Build history of the part. All positions in model axes, mm. Round coordinates to 2 decimals unless told otherwise and drop trailing zeros. Use a Markdown table: item, result.
from build123d import *

# Parameters (mm, degrees)
SKETCH1_W           = 124.35
SKETCH1_H           = 33
BOSS_EXTRUDE1_DEPTH = 3.175
SKETCH2_W           = 9.65
SKETCH2_H           = 2.8
SKETCH2_H_2         = 3
CUT_EXTRUDE1_DEPTH  = 65.405444257
SKETCH4_W           = 2.8
SKETCH4_H           = 3
SKETCH4_W_2         = 6.175
SKETCH4_H_2         = 15
CUT_EXTRUDE2_DEPTH  = 65.405444257
SKETCH6_W           = 3
SKETCH6_H           = 1.375
CUT_EXTRUDE3_DEPTH  = 65.405444257
CUT_SWEEP1_DEPTH    = 3.175
SKETCH12_R          = 0.75
CUT_EXTRUDE6_DEPTH  = 65.405444385
CUT_EXTRUDE7_DEPTH  = 65.405444385
FILLET6_R           = 2
FILLET7_R           = 0.5
SKETCH14_W          = 20
SKETCH14_H          = 16
CUT_EXTRUDE8_DEPTH  = 65.405444385
FILLET8_R           = 0.5


# Read off the part's stored shape, not the designer's step: Cut-Sweep1
with BuildPart() as part:
    # Sketch1 → Boss-Extrude1 (new body)
    with BuildSketch(Plane.XY):
        Rectangle(SKETCH1_W, SKETCH1_H)
    extrude(amount=BOSS_EXTRUDE1_DEPTH)

    # Sketch2 → Cut-Extrude1 (cut, through all)
    with BuildSketch(Plane.XY.offset(3.175)):
        with Locations((-25, -13.1)):
            Rectangle(SKETCH2_W, SKETCH2_H)
        with Locations((25, -13.1)):
            Rectangle(SKETCH2_W, SKETCH2_H)
        with Locations((-25, 15)):
            Rectangle(SKETCH2_W, SKETCH2_H_2)
        with Locations((25, 15)):
            Rectangle(SKETCH2_W, SKETCH2_H_2)
    extrude(amount=-CUT_EXTRUDE1_DEPTH, mode=Mode.SUBTRACT)

    # Sketch4 → Cut-Extrude2 (cut, through all)
    with BuildSketch(Plane.XY.offset(3.175)):
        with Locations((-57.775, 15)):
            Rectangle(SKETCH4_W, SKETCH4_H)
        with Locations((-59.0875, 0)):
            Rectangle(SKETCH4_W_2, SKETCH4_H_2)
        with Locations((-57.775, -15)):
            Rectangle(SKETCH4_W, SKETCH4_H)
        with Locations((57.775, 15)):
            Rectangle(SKETCH4_W, SKETCH4_H)
        with Locations((59.0875, 0)):
            Rectangle(SKETCH4_W_2, SKETCH4_H_2)
        with Locations((57.775, -15)):
            Rectangle(SKETCH4_W, SKETCH4_H)
    extrude(amount=-CUT_EXTRUDE2_DEPTH, mode=Mode.SUBTRACT)

    # Sketch6 → Cut-Extrude3 (cut, through all)
    with BuildSketch(Plane.XY.offset(3.175)):
        with Locations((-60.675, 15.8125)):
            Rectangle(SKETCH6_W, SKETCH6_H)
        with Locations((-60.675, -15.8125)):
            Rectangle(SKETCH6_W, SKETCH6_H)
        with Locations((60.675, 15.8125)):
            Rectangle(SKETCH6_W, SKETCH6_H)
        with Locations((60.675, -15.8125)):
            Rectangle(SKETCH6_W, SKETCH6_H)
    extrude(amount=-CUT_EXTRUDE3_DEPTH, mode=Mode.SUBTRACT)

    # Cut-Sweep1 outline → Cut-Sweep1 (cut)
    with BuildSketch(Plane.XY):
        with BuildLine():
            add(Edge.make_bspline(
                [(-56, -6), (-55.016272395, -6.040912607), (-53.484317245, -6.110006936), (-52.10462272, -6.208217255), (-51.370216858, -6.312882143), (-50.849013323, -6.424427059), (-50.274077583, -6.562740427), (-49.507561658, -6.770408498), (-47.98416767, -7.234467607), (-46.535590196, -7.742954919), (-44.899823838, -8.383891144), (-43.265010906, -9.091671777), (-41.074137026, -10.055384808), (-38.357692762, -10.850187014), (-36.1078612, -11.027108547), (-34.793437631, -10.999002823)],
                knots=[0, 0, 0, 0, 0.052266667, 0.104533333, 0.1568, 0.188540911, 0.209066667, 0.261333333, 0.3136, 0.4368, 0.46346514, 0.56, 0.706666667, 0.853333333, 1, 1, 1, 1], degree=3))
            Line((-56, -6), (-56, -7.5))
            add(Edge.make_bspline(
                [(-56, -7.5), (-55.020423649, -7.540842864), (-53.496771007, -7.609797709), (-52.171479553, -7.70829789), (-51.569513747, -7.80075633), (-51.115986388, -7.900930823), (-50.592043829, -8.028791809), (-49.863497697, -8.22781936), (-48.398796638, -8.676488924), (-46.992197023, -9.172450468), (-45.412650318, -9.7933523), (-43.831176536, -10.480660701), (-41.561928867, -11.478467634), (-38.556226285, -12.350501385), (-36.110914304, -12.525218982), (-34.698750526, -12.49601129)],
                knots=[0, 0, 0, 0, 0.052266667, 0.104533333, 0.1568, 0.188540911, 0.209066667, 0.261333333, 0.3136, 0.4368, 0.46346514, 0.56, 0.706666667, 0.853333333, 1, 1, 1, 1], degree=3))
            Line((-34.698750526, -12.49601129), (-34.793437631, -10.999002823))
        make_face()
    cut_sweep1 = extrude(amount=CUT_SWEEP1_DEPTH, mode=Mode.SUBTRACT)

    # Mirror1: Cut-Sweep1 across plane
    add(cut_sweep1.mirror(Plane.ZY), mode=Mode.SUBTRACT)

    # Sketch12 → Cut-Extrude6 (cut, through all)
    with BuildSketch(Plane.XY.offset(3.175)):
        with Locations((-34.746094079, -11.747507056)):
            Circle(SKETCH12_R)
        with Locations((34.746094079, -11.747507056)):
            Circle(SKETCH12_R)
    extrude(amount=-CUT_EXTRUDE6_DEPTH, mode=Mode.SUBTRACT)

    # Sketch13 → Cut-Extrude7 (cut, through all)
    with BuildSketch(Plane.XY.offset(3.175)):
        Polygon((-56, 7.5), (-62.175, 11.3125), (-62.175, 7.5), align=None)
        Polygon((-56, -7.5), (-62.175, -11.3125), (-62.175, -7.5), align=None)
        Polygon((56, 7.5), (62.175, 11.3125), (62.175, 7.5), align=None)
        Polygon((56, -7.5), (62.175, -11.3125), (62.175, -7.5), align=None)
    extrude(amount=-CUT_EXTRUDE7_DEPTH, mode=Mode.SUBTRACT)

    # Fillet6
    fillet6_edges = [part.edges().sort_by_distance(p)[0] for p in [
        (62.175, -15.125, 1.5875),
        (62.175, -11.3125, 1.5875),
        (56, -7.5, 1.5875),
        (56, 7.5, 1.5875),
        (62.175, 11.3125, 1.5875),
        (62.175, 15.125, 1.5875),
        (-62.175, -15.125, 1.5875),
        (-62.175, -11.3125, 1.5875),
        (-56, -7.5, 1.5875),
        (-62.175, 15.125, 1.5875),
        (-62.175, 11.3125, 1.5875),
        (-56, 7.5, 1.5875),
    ]]
    fillet(fillet6_edges, radius=FILLET6_R)

    # Fillet7
    fillet7_edges = [part.edges().sort_by_distance(p)[0] for p in [
        (59.175, 15.125, 1.5875),
        (59.175, -15.125, 1.5875),
        (-59.175, -15.125, 1.5875),
        (-59.175, 15.125, 1.5875),
        (20.175, 16.5, 1.5875),
        (29.825, 16.5, 1.5875),
        (-20.175, 16.5, 1.5875),
        (-29.825, 16.5, 1.5875),
        (56.375, -16.5, 1.5875),
        (56, -6, 1.5875),
        (56.375, 16.5, 1.5875),
        (-56.375, 16.5, 1.5875),
        (-56.375, -16.5, 1.5875),
        (-56, -6, 1.5875),
    ]]
    fillet(fillet7_edges, radius=FILLET7_R)

    # Sketch14 → Cut-Extrude8 (cut, through all)
    with BuildSketch(Plane.XY.offset(3.175)):
        with Locations((0, 3.275)):
            Rectangle(SKETCH14_W, SKETCH14_H)
    extrude(amount=-CUT_EXTRUDE8_DEPTH, mode=Mode.SUBTRACT)

    # Fillet8
    fillet8_edges = [part.edges().sort_by_distance(p)[0] for p in [
        (-10, -4.725, 1.5875),
        (-10, 11.275, 1.5875),
        (10, 11.275, 1.5875),
        (10, -4.725, 1.5875),
    ]]
    fillet(fillet8_edges, radius=FILLET8_R)


solid = part.part
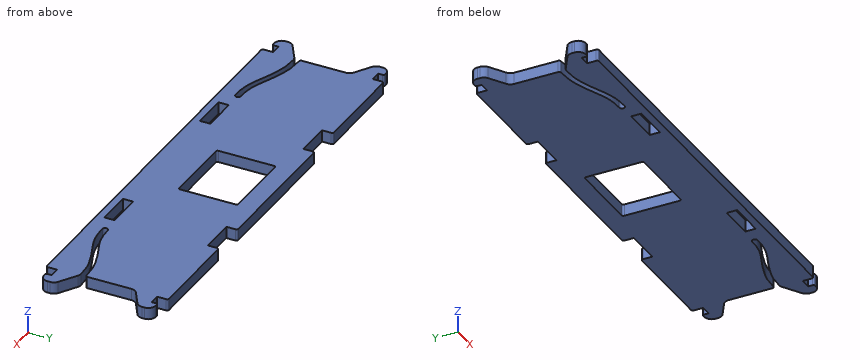
Q1. Drop flat-ended pins along their axis: P1, Ø0.8, axis at y = 14.5, z = 2, coming from the -X side; P2, Ø1.2, axis at y = 14, z = 1.5, coming from the +X side; P3, Ø0.9, axis at y = -14.5, z = 1.5, coming from the +X side. Give the stop position or say it passes through.
Response values:
| item | result |
|---|---|
| P1 | stops at x = -61.92 |
| P2 | stops at x = 62.16 |
| P3 | stops at x = 61.95 |
Q2. Drill centre lines: L1, parallel to X at y = 0, z = 1.2; L2, parallel to Y at x = -22.5, z = 0.8; L3, parallel to Y at x = 0.5, z = 1.45 (3 decimals). Where is each one in solid material? Low to high.
Response values:
| item | result |
|---|---|
| L1 | x = -56 to -10, 10 to 56 |
| L2 | y = -16.5 to -14.5, -11.7 to 13.5 |
| L3 | y = -16.5 to -4.725, 11.275 to 16.5 |
Q3. Cut at A-A on y = -9.5. Count the separate pieces of the cut face and the enclosed holes in it, and give its area (3 significant figures).
Response values:
| item | result |
|---|---|
| separate pieces | 3 |
| enclosed holes | 0 |
| area | 352 mm2 |
